Part model, mm, in its own coordinate system. Round coordinates to 2 decimals unless told otherwise and drop trailing zeros. Write each loop counter-clockwise with the first axis right and the second up, starting at its lowest first coordinate (ties: lowest second). Pieces come first, ordered by that corner, then holes. Notation, with made-up numbers: M 49,34.25 L 71,34.25 A24 cw 71,57.25 Z; hole C -39.75,62 d6. An arc over 180 degrees is marked long. Use a Markdown table: item, result. Add a question column.
1) Slice it at B-B on x = 2. Write the cut outline in (y, z).
2) Drop a flat-ended pin along its axis: P1, Ø2.5, axis at x = 52, y = 35, coming from the -Z side. Give the stop position or say it passes through.
3) Slice it at C-C on x = -35.5. Write the cut outline in (y, z), plus the area to 3 significant figures.
4) Slice it at D-D on y = -12.5. Write the cut outline in (x, z).
5) Slice it at A-A on y = -30.5. Write the cut outline in (x, z).
6) Wall check: probe 1 along X at (y, z) = (-13, 0.05); probe 2 along X at (y, z) = (-40, -0.65); probe 3 along Y at (x, z) = (16, 0.85). Give the ranges that are in metal, low to high.
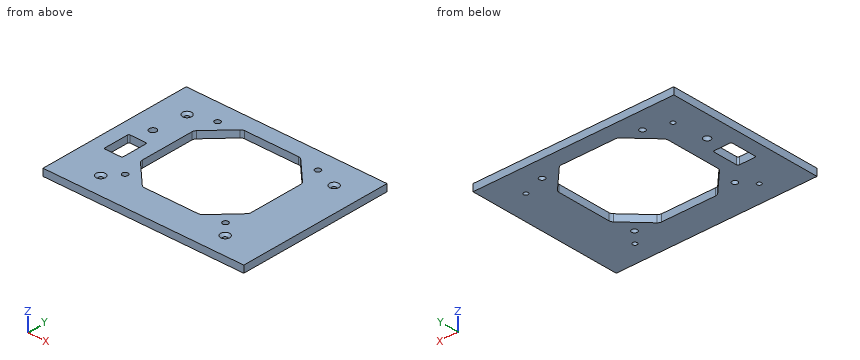
```python
from build123d import *

# Parameters (mm, degrees)
SKETCH1_W                              = 142
SKETCH1_H                              = 110
SHEET_DEPTH                            = 2.5
SKETCH7_R                              = 2
FANHOLES_DEPTH                         = 6
FILLET1_R                              = 3.5
F_3_2_3_2_TOPMOUNTHOLES_D              = 3.2
F_3_2_3_2_TOPMOUNTHOLES_CSINK_D        = 6.5
F_3_2_3_2_TOPMOUNTHOLES_CSINK_ANGLE    = 90
F_3_2_3_2_BOTTOMMOUNTHOLES_D           = 3.2
F_3_2_3_2_BOTTOMMOUNTHOLES_CSINK_D     = 6.5
F_3_2_3_2_BOTTOMMOUNTHOLES_CSINK_ANGLE = 90
SWITCHSLOT_DEPTH                       = 6
SKETCH8_R                              = 2.5
LEDHOLE_DEPTH                          = 6


with BuildPart() as part:
    # Sketch1 → Sheet (new body, symmetric)
    with BuildSketch(Plane.XY):
        Rectangle(SKETCH1_W, SKETCH1_H)
    extrude(amount=SHEET_DEPTH, both=True)

    # Sketch7 → FanHoles (cut, through all)
    with BuildSketch(Plane.XY.offset(2.5)):
        with Locations((-35.5, -30.5)):
            Circle(SKETCH7_R)
        with Locations((35.5, -30.5)):
            Circle(SKETCH7_R)
        with Locations((35.5, 40.5)):
            Circle(SKETCH7_R)
        with Locations((-35.5, 40.5)):
            Circle(SKETCH7_R)
        Polygon((-20.5, 43.5), (-38.5, 25.5), (-38.5, -15.5), (-20.5, -33.5), (20.5, -33.5), (38.5, -15.5), (38.5, 25.5), (20.5, 43.5), align=None)
    extrude(amount=-FANHOLES_DEPTH, mode=Mode.SUBTRACT)

    # Fillet1
    fillet1_edges = [part.edges().sort_by_distance(p)[0] for p in [
        (-20.5, 43.5, 0),
        (20.5, 43.5, 0),
        (38.5, 25.5, 0),
        (38.5, -15.5, 0),
        (20.5, -33.5, 0),
        (-20.5, -33.5, 0),
        (-38.5, -15.5, 0),
        (-38.5, 25.5, 0),
    ]]
    fillet(fillet1_edges, radius=FILLET1_R)

    # Ø3.2 (3.2) TopMountHoles (through all)
    with Locations(Plane.XY.offset(2.5)):
        with Locations((-52, 35), (52, 35)):
            CounterSinkHole(F_3_2_3_2_TOPMOUNTHOLES_D / 2, F_3_2_3_2_TOPMOUNTHOLES_CSINK_D / 2, counter_sink_angle=F_3_2_3_2_TOPMOUNTHOLES_CSINK_ANGLE)

    # Ø3.2 (3.2) BottomMountHoles (through all)
    with Locations(Plane.XY.offset(2.5)):
        with Locations((-44, -40), (44, -40)):
            CounterSinkHole(F_3_2_3_2_BOTTOMMOUNTHOLES_D / 2, F_3_2_3_2_BOTTOMMOUNTHOLES_CSINK_D / 2, counter_sink_angle=F_3_2_3_2_BOTTOMMOUNTHOLES_CSINK_ANGLE)

    # Sketch13 → SwitchSlot (cut, through all)
    with BuildSketch(Plane.XY.offset(2.5)):
        with BuildLine():
            Line((-60, 0), (-49, 0))
            ThreePointArc((-49, 0), (-48.292893219, -0.292893219), (-48, -1))
            Line((-48, -1), (-48, -18.2))
            ThreePointArc((-48, -18.2), (-48.292893219, -18.907106781), (-49, -19.2))
            Line((-49, -19.2), (-60, -19.2))
            ThreePointArc((-60, -19.2), (-60.707106781, -18.907106781), (-61, -18.2))
            Line((-61, -18.2), (-61, -1))
            ThreePointArc((-61, -1), (-60.707106781, -0.292893219), (-60, 0))
        make_face()
    extrude(amount=-SWITCHSLOT_DEPTH, mode=Mode.SUBTRACT)

    # Sketch8 → LEDHole (cut, through all)
    with BuildSketch(Plane.XY.offset(2.5)):
        with Locations((-54.5, 11.5)):
            Circle(SKETCH8_R)
    extrude(amount=-LEDHOLE_DEPTH, mode=Mode.SUBTRACT)


solid = part.part
```
Entries:
| question | item | result |
|---|---|---|
| 1 | outline | M -55,-2.5 L -33.5,-2.5 L -33.5,2.5 L -55,2.5 Z; M 43.5,-2.5 L 55,-2.5 L 55,2.5 L 43.5,2.5 Z |
| 2 | P1 | passes through |
| 3 | outline | M -55,-2.5 L -32.5,-2.5 L -32.5,2.5 L -55,2.5 Z; M -28.5,-2.5 L -18.5,-2.5 L -18.5,2.5 L -28.5,2.5 Z; M 28.5,-2.5 L 38.5,-2.5 L 38.5,2.5 L 28.5,2.5 Z; M 42.5,-2.5 L 55,-2.5 L 55,2.5 L 42.5,2.5 Z |
| 3 | area | 275 mm^2 |
| 4 | outline | M -71,-2.5 L -61,-2.5 L -61,2.5 L -71,2.5 Z; M -48,-2.5 L -38.5,-2.5 L -38.5,2.5 L -48,2.5 Z; M 38.5,-2.5 L 71,-2.5 L 71,2.5 L 38.5,2.5 Z |
| 5 | outline | M -71,-2.5 L -37.5,-2.5 L -37.5,2.5 L -71,2.5 Z; M -33.5,-2.5 L -23.5,-2.5 L -23.5,2.5 L -33.5,2.5 Z; M 23.5,-2.5 L 33.5,-2.5 L 33.5,2.5 L 23.5,2.5 Z; M 37.5,-2.5 L 71,-2.5 L 71,2.5 L 37.5,2.5 Z |
| 6 | probe 1 | x = -71 to -61, -48 to -38.5, 38.5 to 71 |
| 6 | probe 2 | x = -71 to -45.6, -42.4 to 42.4, 45.6 to 71 |
| 6 | probe 3 | y = -55 to -33.5, 43.5 to 55 |
